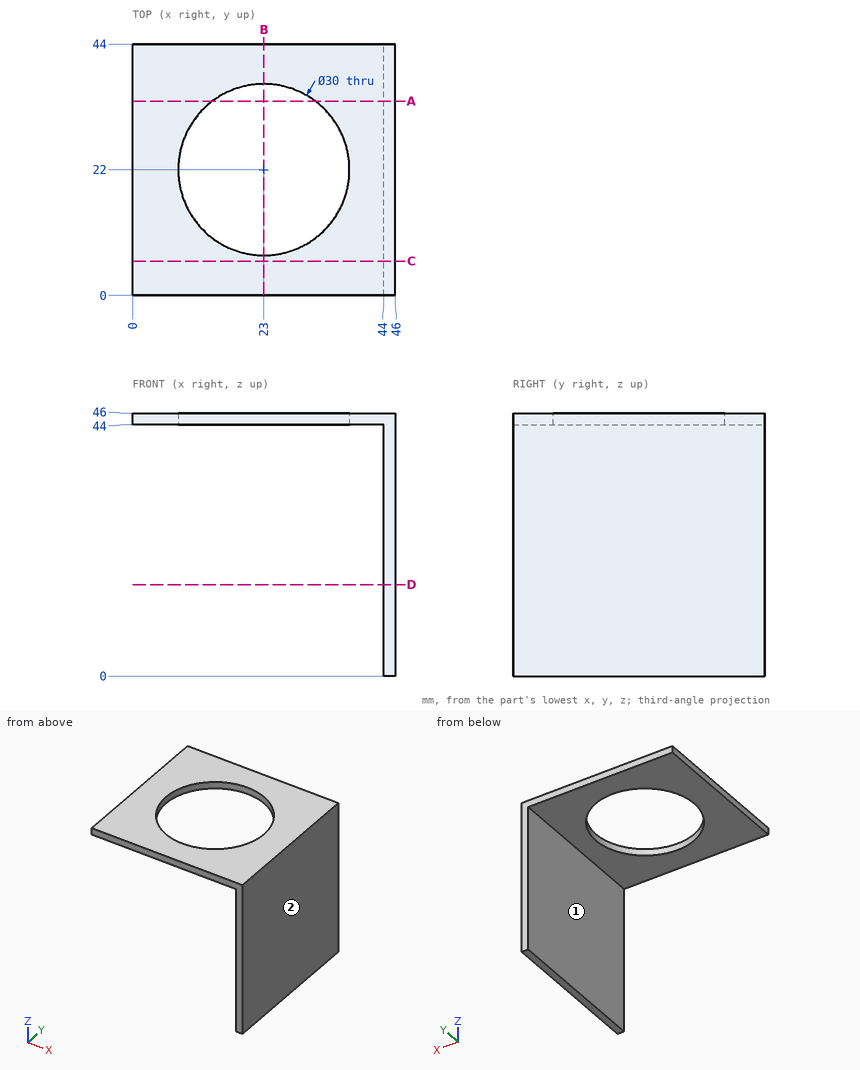
Design review of the part shown in the three views and the two pictorial views. Dimensions are in mm from the part's minimum x, y and z. A direction names the side the tool comes from. Coordinates: 2 decimals unless noted, no trailing zeros. Write each loop counter-clockwise with the first axis right and the second up, starting at its lowest first coordinate (ties: lowest second). Pieces come first, ordered by that corner, then holes.
1) We need section A-A on y = 34. State the section outline as (x, z) points, then the cut area to 3 significant figures.
2) Machinability: for the marked faces 1 and 2, which of the approach directions +Z, -Z, +X, -X, +Y, -Y give a long, thin tool a straight path to every point of the face, cutting with its end or side? Answer none if there is none.
3) We need section B-B on x = 23. State the section outline as (y, z) points.
4) Clearance check with flat-ended pins moving along their axes: pin 1 Ø4 at (x, y) = (8.5, 15) entering from -Z; pin 2 Ø12 at (x, z) = (37.5, 31) entering from +Y; pin 3 Ø6 at (y, z) = (22, 17.5) entering from -X. State where each tip first meets the part, or that it passes through.
5) To check wall thickness, follow probe 1 along X at (y, z) = (22, 45.5); probe 2 along Y at (x, z) = (23, 45.3); probe 3 along X at (y, z) = (22, 29.5). State the ranges of each line that lie inside material, in increasing order.
6) We need section D-D on z = 16. State the section outline as (x, y) points.
7) We need section C-C on y = 6. State the section outline as (x, z) points, then the cut area to 3 significant figures.
Answer list:
1. outline: (0, 44) - (14, 44) - (14, 46) - (0, 46) - close; (32, 44) - (44, 44) - (44, 0) - (46, 0) - (46, 46) - (32, 46) - close
1. area: 144 mm2
2. face 1: -Z, -X, +Y, -Y
2. face 2: +Z, -Z, +X, +Y, -Y
3. outline: (0, 44) - (7, 44) - (7, 46) - (0, 46) - close; (37, 44) - (44, 44) - (44, 46) - (37, 46) - close
4. pin 1: stops at z = 44
4. pin 2: passes through
4. pin 3: stops at x = 44
5. probe 1: x = 0 to 8, 38 to 46
5. probe 2: y = 0 to 7, 37 to 44
5. probe 3: x = 44 to 46
6. outline: (44, 0) - (46, 0) - (46, 44) - (44, 44) - close
7. outline: (0, 44) - (44, 44) - (44, 0) - (46, 0) - (46, 46) - (0, 46) - close
7. area: 180 mm2
